Geometry: final body of the model. Coordinates: model frame, mm. A direction names the side the tool comes from. Round coordinates to 2 decimals unless told otherwise and drop trailing zeros. Loops run counter-clockwise (first coordinate to the right, second up) from the corner with the lowest first, then second, coordinate; pieces in that order, holes last. Notation, with made-up numbers: M 3,79 L 38,79 A32 cw 38,111 Z; hole C 47.25,-34 d5. An arc over 180 degrees is marked long. Return JSON: item names as keys, results as strings.
from build123d import *

# Parameters (mm, degrees)
SKETCH_1_R               = 8.5
EXTRUDE_1_DEPTH          = 15
SKETCH_2_R               = 10
EXTRUDE_2_DEPTH          = 9
SKETCH_3_R               = 1
CUT_EXTRUDE_1_DEPTH      = 10
CUT_EXTRUDE_START        = -2.1
SKETCH_4_R               = 8.5
SKETCH_4_R_2             = 8
CUT_EXTRUDE_2_DEPTH      = 1.4
CHAMFER_1_SIZE           = 0.5
SKETCH_7_R               = 1
CUT_EXTRUDE_3_DEPTH      = 8
PATTERN_CIRCULAR_1_COUNT = 4


with BuildPart() as part:
    # Эскиз1 → Бобышка-Вытянуть1 (new body)
    with BuildSketch(Plane(origin=(0, 0, 0), x_dir=(1, 0, 0), z_dir=(0, 1, 0))):
        with Locations(Location((0, 0, 0), (0, 0, 270))):
            Circle(SKETCH_1_R)
    extrude(amount=EXTRUDE_1_DEPTH)

    # Эскиз2 → Бобышка-Вытянуть2 (add)
    with BuildSketch(Plane(origin=(0, 15, 0), x_dir=(1, 0, 0), z_dir=(0, 1, 0))):
        with Locations(Location((0, 0, 0), (0, 0, 270))):
            Circle(SKETCH_2_R)
    extrude(amount=EXTRUDE_2_DEPTH)

    # Эскиз3 → Вырез-Вытянуть1 (cut)
    with BuildSketch(Plane.XZ):
        with Locations(Location((0, 6, 0), (0, 0, 270))):
            Circle(SKETCH_3_R)
        with Locations(Location((6, 0, 0), (0, 0, 270))):
            Circle(SKETCH_3_R)
        with Locations(Location((0, -6, 0), (0, 0, 270))):
            Circle(SKETCH_3_R)
        with Locations(Location((-6, 0, 0), (0, 0, 270))):
            Circle(SKETCH_3_R)
    extrude(amount=-CUT_EXTRUDE_1_DEPTH, mode=Mode.SUBTRACT)

    # Эскиз4 → Вырез-Вытянуть2 (cut)
    with BuildSketch(Plane.XZ.offset(CUT_EXTRUDE_START)):
        with Locations(Location((0, 0, 0), (0, 0, 270))):
            Circle(SKETCH_4_R)
        with Locations(Location((0, 0, 0), (0, 0, 270))):
            Circle(SKETCH_4_R_2, mode=Mode.SUBTRACT)
    extrude(amount=-CUT_EXTRUDE_2_DEPTH, mode=Mode.SUBTRACT)

    # Фаска1
    chamfer_1_edges = [part.edges().sort_by_distance(p)[0] for p in [
        (0, 0, -8.5),
        (0, 24, -10),
    ]]
    chamfer(chamfer_1_edges, length=CHAMFER_1_SIZE)

    # Эскиз7 → Вырез-Вытянуть3 (cut)
    with BuildSketch(Plane(origin=(6.524591557, 0, 7.578238913), x_dir=(0.7578238912515232, 0, -0.6524591556935956), z_dir=(0.6524591556935956, 0, 0.7578238912515232))):
        with Locations((0, 21)):
            Circle(SKETCH_7_R)
    cut_extrude_3 = extrude(amount=-CUT_EXTRUDE_3_DEPTH, mode=Mode.SUBTRACT)

    # Круговой массив1: Вырез-Вытянуть3 ×4 about axis
    pattern_circular_1_axis = Axis((0, 0, 0), (0, 1, 0))
    for i in range(1, PATTERN_CIRCULAR_1_COUNT):
        add(cut_extrude_3.rotate(pattern_circular_1_axis, i * 360 / PATTERN_CIRCULAR_1_COUNT), mode=Mode.SUBTRACT)


solid = part.part
Q1. Reachability of faces 1 (the flat face through (1.294, 21.014, 1.525)), 2 (the cylindrical face through (8.428, 1.289, -1.107)) from +Z, -Z, +X, -X, +Y, -Y: full face, straight path, thin tool, end or side. Return the list, or none.
Determined:
{"face 1": "none", "face 2": "-Y"}
Q2. Section query C-C (y = 18.75). Output: boundary loops of the cut face in (x, z).
Determined:
{"outline": "C 0,0 d20"}
Q3. Pin query (flat end, axial travel): pin 1 (8 mm diameter, centred on x = -1.5, y = 8.5, fed in from -Z); pin 2 (8 mm diameter, centred on y = 5.5, z = 7.5, fed in from -X); pin 3 (1.2 mm diameter, centred on x = 0, z = 6, fed in from -Y). Return the tip coordinate at first contact, or that it passes through.
Determined:
{"pin 1": "stops at z = -8.5", "pin 2": "stops at x = -7.75", "pin 3": "stops at y = 10"}
Q4. Section query A-A (z = 0). Output: boundary loops of the cut face in (x, y).
Determined:
{"outline": "M -10,15 L -8.5,15 L -8.5,3.5 L -8,3.5 L -8,2.1 L -8.5,2.1 L -8.5,0.5 L -8,0 L -7,0 L -7,10 L -5,10 L -5,0 L 5,0 L 5,10 L 7,10 L 7,0 L 8,0 L 8.5,0.5 L 8.5,2.1 L 8,2.1 L 8,3.5 L 8.5,3.5 L 8.5,15 L 10,15 L 10,23.5 L 9.5,24 L -9.5,24 L -10,23.5 Z"}
Q5. Material intervals for L1, parallel to X at y = 2.5, z = 0; L2, parallel to X at y = 6.5, z = 0; L3, parallel to Y at x = 2.5, z = -9, sorted ascending.
Determined:
{"L1": "x = -8 to -7, -5 to 5, 7 to 8", "L2": "x = -8.5 to -7, -5 to 5, 7 to 8.5", "L3": "y = 15 to 24"}
Q6. Section query B-B (x = 0). Output: boundary loops of the cut face in (y, z).
Determined:
{"outline": "M 0,-8 L 0.5,-8.5 L 2.1,-8.5 L 2.1,-8 L 3.5,-8 L 3.5,-8.5 L 15,-8.5 L 15,-10 L 23.5,-10 L 24,-9.5 L 24,9.5 L 23.5,10 L 15,10 L 15,8.5 L 3.5,8.5 L 3.5,8 L 2.1,8 L 2.1,8.5 L 0.5,8.5 L 0,8 L 0,7 L 10,7 L 10,5 L 0,5 L 0,-5 L 10,-5 L 10,-7 L 0,-7 Z"}
Q7. Section query D-D (x = 2.75). State how many separate pieces and enclosed holes the cut face has, plus the area to 3 significant figures.
Determined:
{"separate pieces": "1", "enclosed holes": "2", "area": "403 mm^2"}
Q8. Pull-direction query (X, two-part tool) for faces 3 (the flat face through (-7.4, 15, -4.5)), 4 (the flat face through (6, 10, 0)), 5 (the cylindrical face through (-7.81, 2.79, 1.73)); classes: pulls with the +X half, pulls with the -X half, needs draft (parallel to the pull), parting line crosses it, or undercut.
Determined:
{"face 3": "needs draft", "face 4": "undercut", "face 5": "parting line crosses it"}
